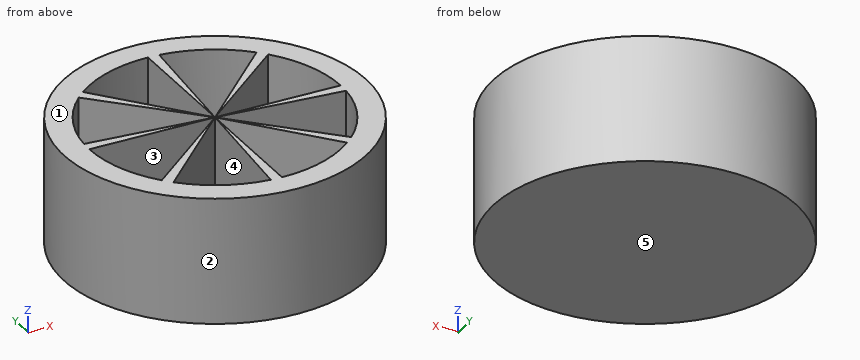
from build123d import *

# Parameters (mm, degrees)
CYLINDER001_W     = 10
CYLINDER001_H     = 12
CYLINDER001_ANGLE = 40
ARRAY_COUNT       = 8
CYLINDER_R        = 12
CYLINDER_DEPTH    = 10


with BuildPart() as array:
    # Cylinder001 → Cylinder001 (revolve)
    with BuildSketch(Plane(origin=(0, 0, 2), x_dir=(1, 0, 0), z_dir=(0, -1, 0))):
        with Locations((5, 6)):
            Rectangle(CYLINDER001_W, CYLINDER001_H)
    revolve(axis=Axis((0, 0, 2), (0, 0, 1)), revolution_arc=CYLINDER001_ANGLE)

    # Array: Array ×8 about axis
    array_axis = Axis((0, 0, 0), (0, 0, 1))


with BuildPart() as array_1:
    add(array.part)
    for i in range(1, ARRAY_COUNT):
        add(array.part.rotate(array_axis, i * 360 / ARRAY_COUNT))


with BuildPart() as cut:
    # Cylinder → Cylinder (new body)
    with BuildSketch(Plane.XY):
        Circle(CYLINDER_R)
    extrude(amount=CYLINDER_DEPTH)

    # Cut: cut Array
    add(array_1.part, mode=Mode.SUBTRACT)


solid = cut.part
Design review of the part built by this model. Coordinates are the model's own, in mm. Face numbers are marked on the shaded views. A direction names the side the tool comes from. Round coordinates to 2 decimals unless told otherwise and drop trailing zeros. Write each loop counter-clockwise with the first axis right and the second up, starting at its lowest first coordinate (ties: lowest second). Pieces come first, ordered by that corner, then holes. Notation, with made-up numbers: (0, 46) -> (28, 46) arc R11 cw to (28, 58) -> close; hole circle Ø4 at (64.5, 33). An arc over 180 degrees is marked (long way). One line per item, written item: value. Start each with the question number.
Q1. To check wall thickness, follow probe 1 along Y at (x, z) = (-7.75, 4.25); probe 2 along X at (y, z) = (7.25, 8); probe 3 along X at (y, z) = (-7.5, 9.75). State the ranges of each line that lie inside material, in increasing order.
Q2. Add section C-C (y = -2). Give the boundary of the cut face in (x, z), then the cut area to 3 significant figures.
Q3. Tool access review of the marked faces 4 and 5: name each direction out of +Z, -Z, +X, -X, +Y, -Y from which nothing blocks a thin tool from reaching the whole face with its end or side.
Q4. Add section B-B (x = 5.5). Give the boundary of the cut face in (y, z), then the cut area to 3 significant figures.
Q5. Add section D-D (z = 1.5). Give the boundary of the cut face in (x, y).
Q6. Insertion check: P1, Ø2, axis at x = -2, z = 2.5, coming from the +Y side; P2, Ø4, axis at y = 6, z = 5.5, coming from the -X side; P3, Ø3, axis at x = 8, y = 4, coming from the -Z side; P4, Ø3, axis at x = 6, y = 2, coming from the +Z side. Each pin has a flat end and moves straight along its axis. Give the tip position at first contact, or say it passes through.
Q7. The part is to be moulded in two halves that separate along Y. For the marked faces 1, 2 and 3, say which applies: pulls with the +Y half, pulls with the -Y half, needs draft (parallel to the pull), parting line crosses it, or undercut.
Response:
1. probe 1: y = -9.16 to -6.32, 0 to 0.68, 6.32 to 9.16
1. probe 2: x = -9.56 to -6.08, 0 to 0.63, 6.89 to 9.56
1. probe 3: x = -9.37 to -6.61, -0.66 to 0, 6.29 to 9.37
2. outline: (-11.83, 0) -> (11.83, 0) -> (11.83, 10) -> (9.8, 10) -> (9.8, 2) -> (2, 2) -> (2, 10) -> (1.68, 10) -> (1.68, 2) -> (0, 2) -> (0, 10) -> (-0.17, 10) -> (-0.17, 2) -> (-2, 2) -> (-2, 10) -> (-2.38, 10) -> (-2.38, 2) -> (-9.8, 2) -> (-9.8, 10) -> (-11.83, 10) -> close
2. area: 86.9 mm^2
3. face 4: +Z
3. face 5: -Z, +X, -X, +Y, -Y
4. outline: (-10.67, 0) -> (10.67, 0) -> (10.67, 10) -> (8.35, 10) -> (8.35, 2) -> (5.5, 2) -> (5.5, 10) -> (4.62, 10) -> (4.62, 2) -> (0, 2) -> (0, 10) -> (-0.48, 10) -> (-0.48, 2) -> (-5.5, 2) -> (-5.5, 10) -> (-6.55, 10) -> (-6.55, 2) -> (-8.35, 2) -> (-8.35, 10) -> (-10.67, 10) -> close
4. area: 99.0 mm^2
5. outline: circle Ø24 at (0, 0)
6. P1: stops at y = 11.96
6. P2: stops at x = -11.31
6. P3: stops at z = 0
6. P4: stops at z = 2
7. face 1: needs draft
7. face 2: parting line crosses it
7. face 3: undercut
